Geometry check sheet. Reference: the model listing, model coordinates, mm. Coordinates: 2 decimals unless noted, no trailing zeros. Loops run counter-clockwise (first coordinate to the right, second up) from the corner with the lowest first, then second, coordinate; pieces in that order, holes last. Notation, with made-up numbers: (35, 1) - (48, 1) arc R25 ccw to (48, 18) - close; hole circle Ø1 at (-39.5, 63.5). An arc over 180 degrees is marked (long way). Write each question's results on one line, items separated by ' | '. Start each with the question number.
(1) Sectioned sample at A-A (x = 6). Enter the section's corners in (y, z), plus the area to 3 significant figures.
(2) Material ranges on probe 1 along Y at (x, z) = (6.75, 1.45); probe 2 along X at (y, z) = (-3.75, 1.75); probe 3 along X at (y, z) = (-4, 1.2), recorded low to high.
(3) Sectioned sample at C-C (y = 2.25). Enter the section's corners in (x, z).
(4) Go/stop test with a flat-tipped pin: pin 1 Ø1.9 at (x, y) = (5.69, -4.52) entering from -Z. Record where the tip stops, or that it passes through.
(5) Sectioned sample at B-B (z = 1.45). State how many separate pieces and enclosed holes the cut face has, plus the area to 3 significant figures.
(6) Sectioned sample at D-D (x = 16.5). Enter the section's corners in (y, z), plus the area to 3 significant figures.
from build123d import *

# Parameters (mm, degrees)
SKETCH1_R           = 3.3782
BOSS_EXTRUDE1_DEPTH = 3.175
SCALE1_SCALE        = 0.35


with BuildPart() as part:
    # Sketch1 → Boss-Extrude1 (new body)
    with BuildSketch(Plane.XY):
        with BuildLine():
            Line((-2.54, 39.37), (2.54, 39.37))
            add(Edge.make_bspline(
                [(2.54, 39.37), (9.095418915, 34.201637521), (9.525, 25.4)],
                knots=[0, 0, 0, 1, 1, 1], degree=2))
            Line((9.525, 25.4), (9.525, 0.833077402))
            Line((9.525, 0.833077402), (13.080713372, -25.725670045))
            Line((13.080713372, -25.725670045), (49.772779476, -31.025635149))
            Line((49.772779476, -31.025635149), (49.772779476, -38.975582805))
            Line((49.772779476, -38.975582805), (10.326960053, -38.975582805))
            Line((10.326960053, -38.975582805), (0, -31.025635149))
            Line((0, -31.025635149), (-9.525, 0))
            Line((-9.525, 0), (-9.525, 25.4))
            add(Edge.make_bspline(
                [(-2.54, 39.37), (-9.095418915, 34.201637521), (-9.525, 25.4)],
                knots=[0, 0, 0, 1, 1, 1], degree=2))
        make_face()
        with Locations((0, 25.4)):
            Circle(SKETCH1_R, mode=Mode.SUBTRACT)
        Circle(SKETCH1_R, mode=Mode.SUBTRACT)
    extrude(amount=BOSS_EXTRUDE1_DEPTH)


with BuildPart() as part_1:
    # Scale1: scaled about (8.755454484, -6.947922753, 1.5875)
    add(part.part.scale(SCALE1_SCALE).moved(Location((5.691045415, -4.516149789, 1.031875))))


solid = part_1.part
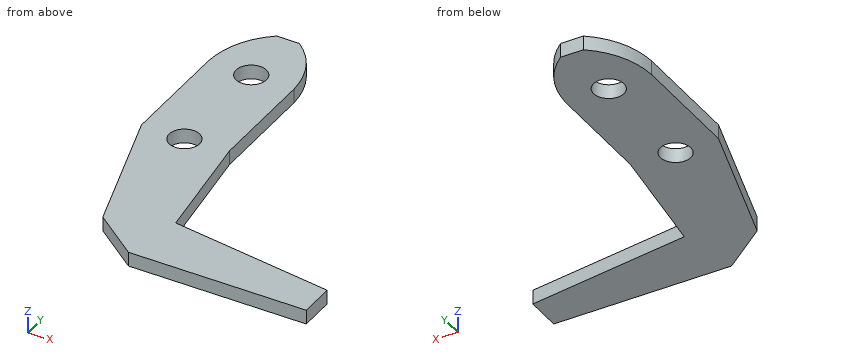
Outcome:
1) outline: (-15.61, 1.03) - (-5.66, 1.03) - (-5.66, 2.14) - (-15.61, 2.14) - close; (-3.37, 1.03) - (3.23, 1.03) - (3.23, 2.14) - (-3.37, 2.14) - close; (5.52, 1.03) - (9.26, 1.03) - (9.26, 2.14) - (5.52, 2.14) - close | area: 22.6 mm2
2) probe 1: y = -16.19 to -5.04, -3.99 to 3.85, 4.9 to 9.13 | probe 2: x = 2.36 to 4.79, 6.59 to 9.02 | probe 3: x = 2.36 to 4.63, 6.75 to 9.02
3) outline: (2.36, 1.03) - (9.02, 1.03) - (9.02, 2.14) - (2.36, 2.14) - close
4) pin 1: passes through
5) separate pieces: 1 | enclosed holes: 2 | area: 193 mm2
6) outline: (-18.16, 1.03) - (-14.42, 1.03) - (-14.42, 2.14) - (-18.16, 2.14) - close | area: 4.15 mm2
